Geometry check sheet. Reference: the model listing, model coordinates, mm. Face numbers are marked on the shaded views. A direction names the side the tool comes from. Give positions to 0.01 mm unless a question says otherwise; leave off trailing zeros. Loops run counter-clockwise (first coordinate to the right, second up) from the corner with the lowest first, then second, coordinate; pieces in that order, holes last.
1. Release check for a two-part mould opening along Z. For the marked faces 1, 2 and 3 record: +Z half, -Z half, draft (parallel to the pull), parting line (faces both ways), or undercut.
2. Cross-section at A-A, the plane x = 0. Record the cut outline in (y, z), plus the area to 3 significant figures.
3. Go/stop test with flat-tipped pins: pin 1 Ø6 at (x, y) = (3, 16) entering from -Z; pin 2 Ø5 at (x, y) = (4, 23.5) entering from -Z; pin 3 Ø6 at (x, y) = (4, 20) entering from +Z; pin 4 Ø1 at (y, z) = (44.5, 1.5) entering from -X. Record where each tip stops, or that it passes through.
4. Tool access check on the marked faces 4 and 5. Record the directions out of +Z, -Z, +X, -X, +Y, -Y that give a thin tool (end or side, any length) a straight path to the whole face; none if there is none.
5. Cross-section at C-C, the plane y = 35. Record the cut outline in (x, z), plus the area to 3 significant figures.
6. Cross-section at B-B, the plane z = 0. Record the cut outline in (x, y).
7. Material ranges on L1, parallel to Z at x = 0, y = 5.5; L2, parallel to Y at x = -1.25, z = 4.75; L3, parallel to X at y = 9, z = -1.75, recorded low to high.
8. Cross-section at D-D, the plane y = 52. Record the cut outline in (x, z).
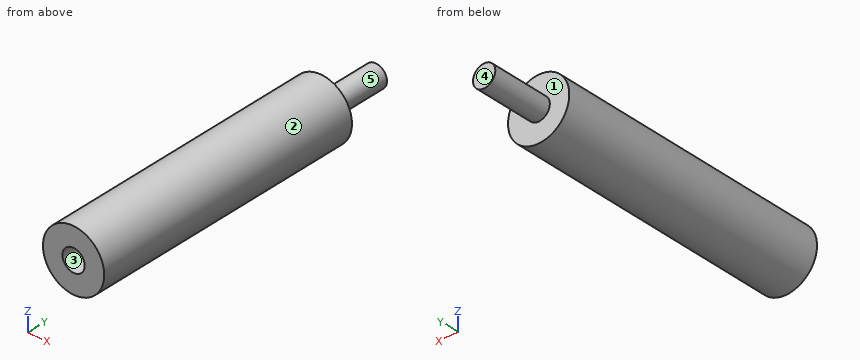
from build123d import *

# Parameters (mm, degrees)
ESQUISSE1_R             = 5.5
BOSS_EXTRU_1_DEPTH      = 50
ESQUISSE2_R             = 2
BOSS_EXTRU_2_DEPTH      = 11
ESQUISSE3_R             = 2
ENL_V_MAT_EXTRU_1_DEPTH = 11


with BuildPart() as part:
    # Esquisse1 → Boss.-Extru.1 (new body)
    with BuildSketch(Plane(origin=(0, 0, 0), x_dir=(1, 0, 0), z_dir=(0, 1, 0))):
        Circle(ESQUISSE1_R)
    extrude(amount=BOSS_EXTRU_1_DEPTH)

    # Esquisse2 → Boss.-Extru.2 (add)
    with BuildSketch(Plane(origin=(0, 50, 0), x_dir=(1, 0, 0), z_dir=(0, 1, 0))):
        Circle(ESQUISSE2_R)
    extrude(amount=BOSS_EXTRU_2_DEPTH)

    # Esquisse3 → Enlèv. mat.-Extru.1 (cut)
    with BuildSketch(Plane.XZ):
        Circle(ESQUISSE3_R)
    extrude(amount=-ENL_V_MAT_EXTRU_1_DEPTH, mode=Mode.SUBTRACT)


solid = part.part
Result:
1. face 1: draft
1. face 2: parting line
1. face 3: undercut
2. outline: (0, -5.5) - (50, -5.5) - (50, -2) - (61, -2) - (61, 2) - (50, 2) - (50, 5.5) - (0, 5.5) - (0, 2) - (11, 2) - (11, -2) - (0, -2) - close
2. area: 550 mm2
3. pin 1: stops at z = -5.5
3. pin 2: stops at z = -5.29
3. pin 3: stops at z = 5.41
3. pin 4: stops at x = -5.41
4. face 4: +Z, -Z, +X, -X, +Y
4. face 5: +Y
5. outline: circle Ø11 at (0, 0)
5. area: 95.0 mm2
6. outline: (-5.5, 0) - (-2, 0) - (-2, 11) - (2, 11) - (2, 0) - (5.5, 0) - (5.5, 50) - (2, 50) - (2, 61) - (-2, 61) - (-2, 50) - (-5.5, 50) - close
7. L1: z = -5.5 to -2, 2 to 5.5
7. L2: y = 0 to 50
7. L3: x = -5.21 to -0.97, 0.97 to 5.21
8. outline: circle Ø4 at (0, 0)
